from build123d import *

# Parameters (mm, degrees)
BOSS_EXTRUDE1_DEPTH = 6
SKETCH2_W           = 7.6
SKETCH2_H           = 8.4
BOSS_EXTRUDE2_DEPTH = 4
SKETCH3_W           = 40
SKETCH3_H           = 30
BOSS_EXTRUDE3_DEPTH = 4
BOSS_EXTRUDE4_DEPTH = 2.5
BOSS_EXTRUDE5_DEPTH = 2.5
FILLET1_R           = 10
SKETCH8_R           = 3
CUT_EXTRUDE1_DEPTH  = 32.2
FILLET2_R           = 1
FILLET3_R           = 0.5
FILLET4_R           = 0.5
FILLET5_R           = 0.5


with BuildPart() as part:
    # Sketch1 → Boss-Extrude1 (new body, symmetric)
    with BuildSketch(Plane(origin=(0, 0, 0), x_dir=(1, 0, 0), z_dir=(0, 1, 0))):
        Polygon((-8, 0), (8, 0), (8, 3.6), (4.3, 7.2), (-4.3, 7.2), (-8, 3.6), align=None)
    extrude(amount=BOSS_EXTRUDE1_DEPTH, both=True)

    # Sketch2 → Boss-Extrude2 (add)
    with BuildSketch(Plane(origin=(0, 0, -7.2), x_dir=(-1, 0, 0), z_dir=(0, 0, -1))):
        Rectangle(SKETCH2_W, SKETCH2_H)
    extrude(amount=BOSS_EXTRUDE2_DEPTH)

    # Sketch3 → Boss-Extrude3 (add)
    with BuildSketch(Plane(origin=(0, 0, -11.2), x_dir=(-1, 0, 0), z_dir=(0, 0, -1))):
        Rectangle(SKETCH3_W, SKETCH3_H)
    extrude(amount=BOSS_EXTRUDE3_DEPTH)

    # Sketch6 → Boss-Extrude4 (add, symmetric)
    with BuildSketch(Plane.ZY.offset(10)):
        Polygon((-27.2, 8), (-15.2, 8), (-15.2, 12), (-31.2, 12), (-31.2, -12), (-23.2, -12), (-23.2, -8), (-27.2, -8), align=None)
    extrude(amount=BOSS_EXTRUDE4_DEPTH, both=True)

    # Sketch7 → Boss-Extrude5 (add, symmetric)
    with BuildSketch(Plane(origin=(10, 0, 0), x_dir=(0, 0, -1), z_dir=(1, 0, 0))):
        Polygon((23.2, 12), (23.2, 8), (27.2, 8), (27.2, -8), (15.2, -8), (15.2, -12), (31.2, -12), (31.2, 12), align=None)
    extrude(amount=BOSS_EXTRUDE5_DEPTH, both=True)

    # Fillet1
    fillet1_edges = [part.edges().sort_by_distance(p)[0] for p in [
        (-20, -15, -13.2),
        (-20, 15, -13.2),
        (20, 15, -13.2),
        (20, -15, -13.2),
    ]]
    fillet(fillet1_edges, radius=FILLET1_R)

    # Sketch8 → Cut-Extrude1 (cut, through all)
    with BuildSketch(Plane.XY):
        Circle(SKETCH8_R)
    extrude(amount=-CUT_EXTRUDE1_DEPTH, mode=Mode.SUBTRACT)

    # Fillet2
    fillet2_edges = [part.edges().sort_by_distance(p)[0] for p in [
        (-3, 0, -15.2),
        (-3, 0, 0),
    ]]
    fillet(fillet2_edges, radius=FILLET2_R)

    # Fillet3
    fillet3_edges = [part.edges().sort_by_distance(p)[0] for p in [
        (-6.15, 6, -5.4),
        (-8, 6, -1.8),
        (0, 6, 0),
        (8, 6, -1.8),
        (6.15, 6, -5.4),
        (8, -6, -1.8),
        (0, -6, 0),
        (-8, -6, -1.8),
        (-6.15, -6, -5.4),
        (0, -6, -7.2),
        (6.15, -6, -5.4),
        (0, 6, -7.2),
    ]]
    fillet(fillet3_edges, radius=FILLET3_R)

    # Fillet4
    fillet4_edges = [part.edges().sort_by_distance(p)[0] for p in [
        (-20, 0, -11.2),
        (-20, 0, -15.2),
        (0, -15, -11.2),
        (20, 0, -11.2),
        (0, 15, -11.2),
        (17.071067812, 12.071067812, -11.2),
        (17.071067812, -12.071067812, -11.2),
        (-17.071067812, 12.071067812, -11.2),
        (-17.071067812, -12.071067812, -11.2),
        (0, -15, -15.2),
        (0, 15, -15.2),
        (20, 0, -15.2),
        (17.071067812, 12.071067812, -15.2),
        (17.071067812, -12.071067812, -15.2),
        (-17.071067812, 12.071067812, -15.2),
        (-17.071067812, -12.071067812, -15.2),
    ]]
    fillet(fillet4_edges, radius=FILLET4_R)

    # Fillet5
    fillet5_edges = [part.edges().sort_by_distance(p)[0] for p in [
        (-3.8, 0, -11.2),
        (0, 4.2, -11.2),
        (3.8, 0, -11.2),
        (0, -4.2, -11.2),
    ]]
    fillet(fillet5_edges, radius=FILLET5_R)


solid = part.part
Geometry check sheet. Reference: the model listing, model coordinates, mm. A direction names the side the tool comes from. Round coordinates to 2 decimals unless told otherwise and drop trailing zeros. Loops run counter-clockwise (first coordinate to the right, second up) from the corner with the lowest first, then second, coordinate; pieces in that order, holes last. Notation, with made-up numbers: (-14, 46) -> (1, 46) arc R13 ccw to (1, 65) -> close; hole circle Ø5 at (-2, 42.5). An arc over 180 degrees is marked (long way). Answer as a JSON object with one key per item and string values. Group by question number.
Item 1: Set-up check for faces 1 (the face through (8, 0, -2)), 2 (the face through (0, -6, -4)), 3 (the face through (-12.5, 3, -29)), 4 (the face through (0, 6, -4)), 5 (the face through (-3.8, 0, -9)): record each of +Z, -Z, +X, -X, +Y, -Y from which the full face is reachable in a straight line by a thin tool's end or side.
Item 2: Depth check by flat-ended pin: pin 1 Ø13 at (y, z) = (-5.5, -20.5) entering from +X; pin 2 Ø1.7 at (y, z) = (0.5, -9) entering from +X; pin 3 Ø4 at (y, z) = (-3.5, -27.5) entering from -X; pin 4 Ø10 at (x, z) = (10, -21.5) entering from +Y. Enter the tip coordinate at first touch or a pass-through.
Item 3: Cross-section at A-A, the plane z = -16.5. Record the cut outline in (x, y).
Item 4: Release check for a two-part mould opening along Z. For faces 6 (the face through (10, 10, -23.2)), 7 (the face through (6.18, 0.08, -5.37)), 8 (the face through (10, 0, -31.2)), 9 (the face through (-7.5, 3, -29)) record: pulls with the +Z half, pulls with the -Z half, needs draft (parallel to the pull), parting line crosses it, or undercut.
Item 5: Thickness scan on line 1 along Y through (x, z) = (0, -8); line 2 along Y through (x, z) = (0, -5); line 3 along X through (y, z) = (9, -24). Record the ranges inside material, lowest first.
Item 6: Cross-section at C-C, the plane x = -8.5. Record the cut outline in (y, z), plus the area to 3 significant figures.
Item 7: Cross-section at D-D, the plane y = 0. Count the separate pieces of the cut face and the enclosed holes in it, plus the area to 3 significant figures.
Determined:
{
 "1": {"face 1": "+Z, +X, +Y, -Y", "face 2": "+Z, +X, -X, -Y", "face 3": "-Z, -X, +Y, -Y", "face 4": "+Z, +X, -X, +Y", "face 5": "-X, +Y, -Y"},
 "2": {"pin 1": "stops at x = 20", "pin 2": "stops at x = 3.8", "pin 3": "stops at x = -12.5", "pin 4": "stops at y = 12"},
 "3": {"outline": "(-12.5, 8) -> (-7.5, 8) -> (-7.5, 12) -> (-12.5, 12) -> close; (7.5, -12) -> (12.5, -12) -> (12.5, -8) -> (7.5, -8) -> close"},
 "4": {"face 6": "undercut", "face 7": "undercut", "face 8": "pulls with the -Z half", "face 9": "needs draft"},
 "5": {"line 1": "y = -4.2 to -3, 3 to 4.2", "line 2": "y = -6 to -3, 3 to 6", "line 3": "x = -12.5 to -7.5, 7.5 to 12.5"},
 "6": {"outline": "(-15, -14.7) arc R0.5 ccw to (-14.5, -15.2) -> (8, -15.2) -> (8, -27.2) -> (-8, -27.2) -> (-8, -23.2) -> (-12, -23.2) -> (-12, -31.2) -> (12, -31.2) -> (12, -15.2) -> (14.5, -15.2) arc R0.5 ccw to (15, -14.7) -> (15, -11.7) arc R0.5 ccw to (14.5, -11.2) -> (-14.5, -11.2) arc R0.5 ccw to (-15, -11.7) -> close", "area": "280 mm²"},
 "7": {"separate pieces": "4", "enclosed holes": "0", "area": "240 mm²"}
}
